Geometry check sheet. Reference: the model listing, model coordinates, mm. A direction names the side the tool comes from. Give positions to 0.01 mm unless a question says otherwise; leave off trailing zeros. Loops run counter-clockwise (first coordinate to the right, second up) from the corner with the lowest first, then second, coordinate; pieces in that order, holes last. Notation, with made-up numbers: (60.25, 64) -> (93.25, 64) arc R31 cw to (93.25, 89) -> close; hole circle Ø10 at (-24.5, -18.5). An arc over 180 degrees is marked (long way). Write item = value, one per line.
Autodesk Inventor part; units mm, degrees
ref_plane "YZ Plane" through (0, 0, 0) normal (1, 0, 0) x (0, 1, 0)
ref_plane "XZ Plane" through (0, 0, 0) normal (0, 1, 0) x (-1, 0, 0)
ref_plane "XY Plane" through (0, 0, 0) normal (0, 0, 1) x (1, 0, 0)
sketch "Sketch1" plane through (0, 0, 0) normal (0, 1, 0) x (-1, 0, 0)
  line L0 (69.5314, 72.8452) -> (-57.4686, 72.8452)
  line L1 (-57.4686, 72.8452) -> (-57.4686, 32.2052)
  line L2 (-57.4686, 32.2052) -> (69.5314, 32.2052)
  line L3 (69.5314, 32.2052) -> (69.5314, 72.8452)
  point P0 (0, 0)
  dimension "d0" = 127
  dimension "d1" = 40.64
extrude "Extrusion1" add sketch "Sketch1" along normal blind 6.35
sketch "Sketch2" plane through (0, 6.35, 0) normal (0, 1, 0) x (1, 0, 0)
  line L0 (-50.2274, -32.2052) -> (38.4186, -32.2052)
  line L1 (38.4186, -32.2052) -> (38.4186, -72.8452)
  line L2 (38.4186, -72.8452) -> (-50.2274, -72.8452)
  line L3 (-50.2274, -72.8452) -> (-50.2274, -32.2052)
  line L4 (-69.5314, -32.2052) -> (-69.5314, -72.8452)
  line L5 (57.4686, -72.8452) -> (57.4686, -32.2052)
  line L6 (57.4686, -32.2052) -> (-69.5314, -32.2052)
  line L7 (-69.5314, -72.8452) -> (57.4686, -72.8452)
  point P0 (0, 0)
  dimension "d4" = 19.304
  dimension "d5" = 19.05
  dimension "d6" = 0
  dimension "d7" = 0
extrude "Extrusion2" add sketch "Sketch2" along normal blind 6.35 contours L0 L1 L2 L3
sketch "Sketch3" plane through (0, 6.35, 0) normal (0, 1, 0) x (1, 0, 0)
  line L0 (57.4686, -32.2052) -> (38.4186, -32.2052)
  line L1 (57.4686, -72.8452) -> (57.4686, -32.2052)
  line L2 (-69.5314, -32.2052) -> (-69.5314, -72.8452)
  line L3 (-50.2274, -32.2052) -> (-69.5314, -32.2052)
  line L4 (-69.5314, -72.8452) -> (-50.2274, -72.8452)
  line L5 (38.4186, -72.8452) -> (57.4686, -72.8452)
  circle A0 centre (-27.5338, -49.4612) radius 4.3448
  circle A1 centre (16.1358, -48.3961) radius 3.4084
  point P0 (0, 0)
  point P1 (-56.8314, -44.9052)
  point P2 (-56.8314, -60.1452)
  point P3 (44.7686, -44.9052)
  point P4 (44.7686, -60.1452)
  dimension "d10" = 12.7
  dimension "d11" = 12.7
  dimension "d12" = 12.7
  dimension "d13" = 12.7
  dimension "d14" = 12.7
  dimension "d15" = 12.7
  dimension "d16" = 12.7
  dimension "d17" = 12.7
hole "Hole1" at (-56.8314, 6.35, 44.9052) at (-56.8314, 6.35, 60.1452) at (44.7686, 6.35, 44.9052) at (44.7686, 6.35, 60.1452) direction (0, -1, 0) diameter 5.1054 depth 25.4 tip angle 118
sketch "Sketch4" plane through (0, 0, 0) normal (0, -1, 0) x (1, 0, 0)
  circle A0 centre (-18.7314, 52.5252) radius 4.445
  circle A1 centre (6.6686, 52.5252) radius 4.445
  line L0 (57.4686, 32.2052) -> (-69.5314, 32.2052)
  line L1 (57.4686, 72.8452) -> (57.4686, 32.2052)
  line L2 (-69.5314, 32.2052) -> (-69.5314, 72.8452)
  point P0 (0, 0)
  dimension "d25" = 20.32
  dimension "d26" = 0
  dimension "d27" = 50.8
  dimension "d28" = 50.8
  dimension "d29" = 8.89
  dimension "d30" = 8.89
extrude "Extrusion3" cut sketch "Sketch4" against normal blind 7.62
sketch "Sketch5" plane through (0, 0, 0) normal (0, -1, 0) x (1, 0, 0)
  point P0 (0, 0)
sketch "Sketch6" plane through (0, 0, 0) normal (0, -1, 0) x (1, 0, 0)
  circle A0 centre (-18.7314, 52.5252) radius 4.445
  circle A1 centre (6.6686, 52.5252) radius 4.445
  point P0 (0, 0)
hole "Hole2" at (-18.7314, 0, 52.5252) at (6.6686, 0, 52.5252) direction (0, 1, 0) diameter 4.4958 depth 25.4 tip angle 118
properties part number "HandleBlock"
Item 1: Section check B-B, the plane z = 59.5. Record the cut outline in (x, y).
Answer:
outline = (-69.53, 0) -> (-59.3, 0) -> (-59.3, 6.35) -> (-69.53, 6.35) -> close; (-54.36, 0) -> (42.3, 0) -> (42.3, 6.35) -> (38.42, 6.35) -> (38.42, 12.7) -> (-50.23, 12.7) -> (-50.23, 6.35) -> (-54.36, 6.35) -> close; (47.24, 0) -> (57.47, 0) -> (57.47, 6.35) -> (47.24, 6.35) -> close
Item 2: Section check D-D, the plane y = 10.75. Record the cut outline in (x, z).
Answer:
outline = (-50.23, 32.21) -> (38.42, 32.21) -> (38.42, 72.85) -> (-50.23, 72.85) -> close; hole circle Ø4.5 at (-18.73, 52.53); hole circle Ø4.5 at (6.67, 52.53)
Item 3: Gauge pin test, flat ends, axial feed: pin 1 (4.5 mm diameter, centred on x = 44.77, z = 44.91, fed in from -Y); pin 2 (6.5 mm diameter, centred on x = 44.77, z = 60.15, fed in from +Y); pin 3 (3 mm diameter, centred on y = 9.5, z = 53, fed in from -X); pin 4 (7 mm diameter, centred on x = -18.73, z = 52.53, fed in from -Y). Record the tip position at first contact, or that the pin passes through.
Answer:
pin_1 = through
pin_2 = 6.35
pin_3 = -50.23
pin_4 = 7.62
Item 4: Section check C-C, the plane y = 2. Record the cut outline in (x, z) (3 decimals).
Answer:
outline = (-69.531, 32.205) -> (57.469, 32.205) -> (57.469, 72.845) -> (-69.531, 72.845) -> close; hole circle Ø5.105 at (-56.831, 44.905); hole circle Ø5.105 at (-56.831, 60.145); hole circle Ø8.89 at (-18.731, 52.525); hole circle Ø8.89 at (6.669, 52.525); hole circle Ø5.105 at (44.769, 44.905); hole circle Ø5.105 at (44.769, 60.145)
Item 5: Thickness scan on L1, parallel to X at y = 1.25, z = 53; L2, parallel to Y at x = 40, z = 55; L3, parallel to X at y = 9.75, z = 67. Record the ranges inside material, lowest first. Write a range as [from, to].
Answer:
L1 = [-69.53, -23.15], [-14.31, 2.25], [11.09, 57.47]
L2 = [0, 6.35]
L3 = [-50.23, 38.42]
Item 6: Section check A-A, the plane z = 65. Record the cut outline in (x, y), plus the area to 3 significant figures.
Answer:
outline = (-69.53, 0) -> (57.47, 0) -> (57.47, 6.35) -> (38.42, 6.35) -> (38.42, 12.7) -> (-50.23, 12.7) -> (-50.23, 6.35) -> (-69.53, 6.35) -> close
area = 1,370 mm^2
Item 7: Draft check along X on faces 1 (the flat face through (-5, 6, 32.205)), 2 (the flat face through (38.419, 9, 52)), 3 (the cylindrical face through (6.57, 10.2, 54.77)). Enter one of: +X half, -X half, draft (parallel to the pull), parting line (faces both ways), or undercut.
Answer:
face_1 = draft
face_2 = +X half
face_3 = undercut
Item 8: Tool access check on faces 4 (the flat face through (6, 7.62, 55)), 5 (the flat face through (-5, 0, 53)), 6 (the flat face through (-50.227, 9, 53)), 7 (the flat face through (-69.531, 3, 52)), 8 (the flat face through (48, 6.35, 53)). Record the directions out of +Z, -Z, +X, -X, +Y, -Y that give a thin tool (end or side, any length) a straight path to the whole face; none if there is none.
Answer:
face_4 = -Y
face_5 = +Z, -Z, +X, -X, -Y
face_6 = +Z, -Z, -X, +Y
face_7 = +Z, -Z, -X, +Y, -Y
face_8 = +Z, -Z, +X, +Y
